```python
from build123d import *

# Parameters (mm, degrees)
F2_R     = 1.27
F4_DEPTH = 12.7
F6_DEPTH = 127
F7_SIZE  = 0.254


with BuildPart() as f1:
    # F0 (on Front) → F1 (revolve)
    with BuildSketch(Plane.XZ):
        Polygon((-67.31, 0), (0, 0), (0, 1.2), (-41.9735, 1.2), (-41.9735, 13.9), (-67.31, 3.81), align=None)
    revolve(axis=Axis((0, 0, 6.192707), (0, 0, -1)))

    # F2
    f2_edges = [f1.edges().sort_by_distance(p)[0] for p in [
        (67.31, 0, 3.81),
    ]]
    fillet(f2_edges, radius=F2_R)

    # F3 (on face) → F4 (join)
    with BuildSketch(Plane.XY.offset(1.2)):
        with BuildLine():
            ThreePointArc((-2.4765, 28.110855), (-5.068633, 33.22954), (-10.728763, 34.169229))
            ThreePointArc((-10.728763, 34.169229), (-27.279607, 23.204862), (-35.447604, 5.10979))
            Line((-35.447604, 5.10979), (-31.59345, 5.10979))
            ThreePointArc((-31.59345, 5.10979), (-24.511453, 20.577772), (-10.503515, 30.231311))
            ThreePointArc((-10.503515, 30.231311), (-7.621361, 29.819549), (-6.2865, 27.232173))
            Line((-6.2865, 27.232173), (-6.2865, 18.455401))
            Line((-6.2865, 18.455401), (-2.4765, 18.455401))
            Line((-2.4765, 18.455401), (-2.4765, 28.110855))
        make_face()
        with BuildLine():
            ThreePointArc((-35.447604, -5.10979), (-27.279607, -23.204862), (-10.728763, -34.169229))
            ThreePointArc((-10.728763, -34.169229), (-5.068633, -33.22954), (-2.4765, -28.110855))
            Line((-2.4765, -28.110855), (-2.4765, -18.455401))
            Line((-2.4765, -18.455401), (-6.2865, -18.455401))
            Line((-6.2865, -18.455401), (-6.2865, -27.232173))
            ThreePointArc((-6.2865, -27.232173), (-7.621361, -29.819549), (-10.503515, -30.231311))
            ThreePointArc((-10.503515, -30.231311), (-24.511453, -20.577772), (-31.59345, -5.10979))
            Line((-31.59345, -5.10979), (-35.447604, -5.10979))
        make_face()
    extrude(amount=F4_DEPTH)

    # F5 (on Right) → F6 (cut)
    with BuildSketch(Plane.YZ):
        with BuildLine():
            Line((2.8575, 13.9), (-2.8575, 13.9))
            Line((-2.8575, 13.9), (-2.8575, 7.7405))
            ThreePointArc((-2.8575, 7.7405), (0, 4.883), (2.8575, 7.7405))
            Line((2.8575, 7.7405), (2.8575, 13.9))
        make_face()
    extrude(amount=-F6_DEPTH, mode=Mode.SUBTRACT)

    # F7
    f7_edges = [f1.edges().sort_by_distance(p)[0] for p in [
        (67.31, 0, 0),
    ]]
    chamfer(f7_edges, length=F7_SIZE)


solid = f1.part
```
Input: part model. Units: mm. Frame: model coordinates. A direction names the side the tool comes from. Coordinates: 2 decimals unless noted, no trailing zeros. One line per item, written item: value.
(1) Pull-direction query (X, two-part tool) for faces 4 (the cylindrical face through (14.59, -65.71, 1.58)), 5 (the cylindrical face through (-7.587, -29.795, 7.461)), 6 (the flat face through (-20, -26, 13.9)); classes: +X half, -X half, draft (parallel to the pull), parting line (faces both ways), or undercut.
Filled in:
face 4: parting line
face 5: undercut
face 6: draft
(2) Line query: line 1 along X through (y, z) = (6.5, 3.5); line 2 along Z through (x, y) = (-37, 44); line 3 along Y through (x, z) = (-33, 2). Output: solid intervals per line, ascending. Write a range as from..to.
Filled in:
line 1: -66.87..-41.47, -35.22..-31.34, 41.47..66.87
line 2: 0..7.72
line 3: -58.67..-25.94, -13.92..-5.11, 5.11..13.92, 25.94..58.67
(3) Reachability of faces 1 (the flat face through (-33, -5.11, 7)), 2 (the flat face through (-48, -2.858, 10)), 3 (the flat face through (1, 1, 0)) from +Z, -Z, +X, -X, +Y, -Y: full face, straight path, thin tool, end or side. Return the list, or none.
Filled in:
face 1: +Z
face 2: +Z, -X
face 3: -Z, +X, -X, +Y, -Y
(4) Pin query (flat end, axial travel): pin 1 (5 mm diameter, centred on x = 8, y = 2.5, fed in from +Z); pin 2 (7 mm diameter, centred on y = 24.5, z = 7.5, fed in from -X); pin 3 (5 mm diameter, centred on x = 35.5, z = 2, fed in from -Y). Return the tip coordinate at first contact, or that it passes through.
Filled in:
pin 1: z = 1.2
pin 2: x = -62.24
pin 3: y = -58.67
(5) Section A-A (z = 10). Give the number of separate pieces and of enclosed holes in the cut face, and give its area (3 significant figures).
Filled in:
separate pieces: 3
enclosed holes: 0
area: 3,260 mm^2
